Part model, mm, in its own coordinate system. Face numbers are marked on the shaded views. Give positions to 0.01 mm unless a question says otherwise; leave off trailing zeros. Order: outer loops, then holes, each group sorted by start corner. A loop starts at its lowest first (then second) coordinate and runs counter-clockwise, first axis right, second up. Notation, with made-up numbers: (49, -6.75) - (65, -6.75) arc R22 cw to (65, -0.75) - close; hole circle Ø4 at (12, 48). An arc over 180 degrees is marked (long way). Use one line per item in the form item = value. Start each with the question number.
1. Band-saw the part on C-C, the plane z = 243.5. List the corners of the cut face in (x, y), plus the area to 3 significant figures.
2. Band-saw the part on A-A, the plane x = 0. List the corners of the cut face in (y, z), plus the area to 3 significant figures.
3. Pull direction X, two halves, no side cores. Call the marked faces 1 and 2: +X half, -X half, draft (parallel to the pull), parting line (faces both ways), or undercut.
4. Pin check, flat tips, straight feed: P1, Ø1, axis at y = 1.5, z = 234, coming from the +X side; P2, Ø1, axis at x = -3.5, z = 229.5, coming from the -Y side. Stop position of each tip, or through.
5. Band-saw the part on B-B, the plane z = 236.25. List the corners of the cut face in (x, y), plus the area to 3 significant figures.
6. Drill centre lines: line 1 (X direction, y = 0.5, z = 236.25); line 2 (Z direction, x = 13, y = 0.65); line 3 (X direction, y = 1.45, z = 233.5). Where is each one in solid material? Low to high.
7. Band-saw the part on D-D, the plane z = 232.75. List the corners of the cut face in (x, y).
from build123d import *

# Parameters (mm, degrees)
SKETCH2_R           = 2.650000000000004
BOSS_EXTRUDE1_DEPTH = 2
BOSS_EXTRUDE2_DEPTH = 2
CHAMFER1_SIZE       = 4
CHAMFER1_SIZE2      = 0.5621633388095701


with BuildPart() as part:
    # Sketch2 → Boss-Extrude1 (new body)
    with BuildSketch(Plane(origin=(0, 0, 0), x_dir=(1, 0, 0), z_dir=(0, 1, 0))):
        with BuildLine():
            Line((-15.984695958466673, -228.5918021170437), (-17.33448372541018, -247.89466648957097))
            ThreePointArc((-17.33448372541018, -247.89466648957097), (4.98147e-12, -248.50000000000463), (17.334483725420203, -247.89466648957094))
            Line((17.334483725420203, -247.89466648957094), (15.98469595846676, -228.59180211704373))
            ThreePointArc((15.98469595846676, -228.59180211704373), (4.411e-14, -229.150000000005), (-15.984695958466673, -228.5918021170437))
        make_face()
        with Locations(Location((8.9e-16, -236.24999999999997, 0), (0, 0, 270))):
            Circle(SKETCH2_R, mode=Mode.SUBTRACT)
    extrude(amount=BOSS_EXTRUDE1_DEPTH)

    # Sketch3 → Boss-Extrude2 (add)
    with BuildSketch(Plane(origin=(0, 0, 0), x_dir=(1, 0, 0), z_dir=(0, 1, 0))):
        with BuildLine():
            Line((-15.70567006349017, -224.6015459160044), (-15.984695958466673, -228.5918021170437))
            ThreePointArc((-15.984695958466673, -228.5918021170437), (1.403e-14, -229.15000000000495), (15.98469595846676, -228.59180211704367))
            Line((15.98469595846676, -228.59180211704367), (15.705670063490256, -224.60154591600437))
            ThreePointArc((15.705670063490256, -224.60154591600437), (1.379e-14, -225.15000000000495), (-15.70567006349017, -224.6015459160044))
        make_face()
    extrude(amount=BOSS_EXTRUDE2_DEPTH)

    # Chamfer1
    chamfer1_edges = [part.edges().sort_by_distance(p)[0] for p in [
        (4.53e-14, 0, 225.15000000000498),
    ]]
    chamfer1_side = [part.faces().sort_by_distance(p)[0] for p in [
        (5.01431e-12, 0, 248.07892121738644),
    ]]
    chamfer(chamfer1_edges, length=CHAMFER1_SIZE, length2=CHAMFER1_SIZE2, reference=chamfer1_side[0])


solid = part.part
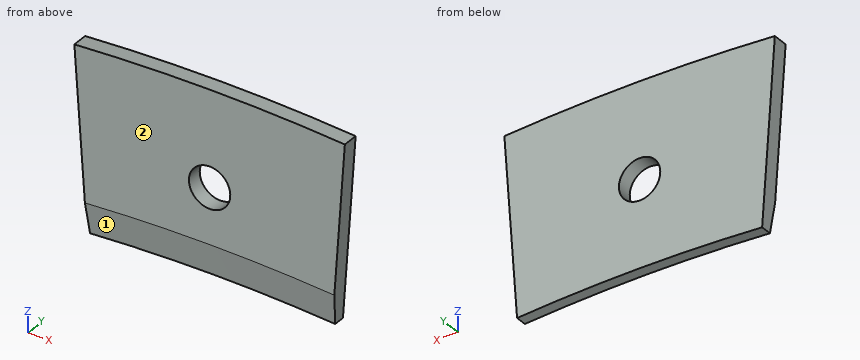
From the geometry:
q1.outline = (-17.03, 0) - (17.03, 0) - (17.03, 2) - (-17.03, 2) - close
q1.area = 68.1 mm²
q2.outline = (0, 229.15) - (0.56, 225.15) - (2, 225.15) - (2, 233.6) - (0, 233.6) - close; (0, 238.9) - (2, 238.9) - (2, 248.5) - (0, 248.5) - close
q2.area = 35.0 mm²
q3.face_1 = undercut
q3.face_2 = draft
q4.P1 = 16.4
q4.P2 = 0
q5.outline = (-16.52, 0) - (-2.65, 0) - (-2.65, 2) - (-16.52, 2) - close; (2.65, 0) - (16.52, 0) - (16.52, 2) - (2.65, 2) - close
q5.area = 55.5 mm²
q6.line_1 = -16.52 to -2.65, 2.65 to 16.52
q6.line_2 = 224.77 to 248.16
q6.line_3 = -16.33 to 16.33
q7.outline = (-16.28, 0) - (16.28, 0) - (16.28, 2) - (-16.28, 2) - close
